The listing builds one solid part. Answer for the finished solid, in the listing's coordinates (mm). Face numbers are marked on the shaded views. A direction names the side the tool comes from. Round coordinates to 2 decimals unless told otherwise and drop trailing zeros. Order: outer loops, then holes, each group sorted by start corner. A loop starts at its lowest first (then second) coordinate and runs counter-clockwise, first axis right, second up. Notation, with made-up numbers: M 80.5,70.5 L 117.5,70.5 A27 cw 117.5,109.5 Z; hole C 12,44.25 d3. An arc over 180 degrees is marked long. Put each result on its own line as item: value. Start each with the question number.
1. The part is cut by section A-A (x = -8.5). Give the vertices of the cut face in (y, z).
2. The part is cut by section D-D (z = 2). Give the vertices of the cut face in (x, y), then the cut area to 3 significant figures.
3. Which of the six approach directions +Z, -Z, +X, -X, +Y, -Y give full straight-line access (tool end or side, diameter ignored) to the marked faces 1, 2, 3 and 4?
4. The part is cut by section C-C (x = -32). Give the vertices of the cut face in (y, z).
5. Each of these flat-tipped pins is pushed along its axis until it touches: pin 1 Ø6 at (x, y) = (-6.5, 62.5) entering from -Z; pin 2 Ø4.5 at (x, z) = (40, -12.5) entering from +Y; pin 3 Ø2 at (x, y) = (-1, -39) entering from -Z. Where does it stop, or does it pass through?
6. Consider line 1 (X direction, y = -82, z = 19); line 2 (Y direction, x = 36, z = 19.3); line 3 (Y direction, x = 15, z = 12.5). Determine where each line is inside the solid, lowest interval first.
7. The part is cut by section B-B (y = -38). Give the vertices of the cut face in (x, z), then the cut area to 3 significant figures.
8. The mould has two halves that part along Y. Classify the marked faces 5, 6 and 7: +Y half, -Y half, draft (parallel to the pull), parting line (faces both ways), or undercut.
from build123d import *

# Parameters (mm, degrees)
SKETCH1_W           = 75
SKETCH1_H           = 168
BOSS_EXTRUDE1_DEPTH = 20
BOSS_EXTRUDE2_DEPTH = 10
SKETCH3_W           = 6
SKETCH3_H           = 6
CUT_EXTRUDE2_DEPTH  = 39.37
SKETCH6_W           = 4
SKETCH6_H           = 5
CUT_EXTRUDE4_DEPTH  = 5
SKETCH7_W           = 69
SKETCH7_H           = 131
CUT_EXTRUDE5_DEPTH  = 16
SKETCH8_W           = 68.924591969
SKETCH8_H           = 27.4
CUT_EXTRUDE6_DEPTH  = 16
SKETCH9_W           = 16
SKETCH9_H           = 8
CUT_EXTRUDE7_DEPTH  = 16
SKETCH11_W          = 7.457157679
SKETCH11_H          = 6
CUT_EXTRUDE8_DEPTH  = 16
BOSS_EXTRUDE3_DEPTH = 10
FILLET4_START       = -3
FILLET4_DEPTH       = 6
FILLET4_START_2     = -50
FILLET4_2_DEPTH     = 131
FILLET5_R           = 2.2
SKETCH13_W          = 7
SKETCH13_H          = 18
BOSS_EXTRUDE4_DEPTH = 8
SKETCH14_W          = 2
SKETCH14_H          = 12.5
CUT_EXTRUDE9_DEPTH  = 99.169037889
SKETCH15_W          = 2
SKETCH15_H          = 12.5
CUT_EXTRUDE10_DEPTH = 99.169037889
SKETCH17_R          = 1
CUT_EXTRUDE11_DEPTH = 2


with BuildPart() as part:
    # Sketch1 → Boss-Extrude1 (new body)
    with BuildSketch(Plane.XY):
        Rectangle(SKETCH1_W, SKETCH1_H)
    extrude(amount=BOSS_EXTRUDE1_DEPTH)

    # Sketch7 → Cut-Extrude5 (cut)
    with BuildSketch(Plane.XY.offset(20)):
        with Locations((0, 15.5)):
            Rectangle(SKETCH7_W, SKETCH7_H)
    extrude(amount=-CUT_EXTRUDE5_DEPTH, mode=Mode.SUBTRACT)

    # Sketch8 → Cut-Extrude6 (cut)
    with BuildSketch(Plane.XY.offset(20)):
        with Locations((-0.037704015, -66.7)):
            Rectangle(SKETCH8_W, SKETCH8_H)
    extrude(amount=-CUT_EXTRUDE6_DEPTH, mode=Mode.SUBTRACT)

    # Sketch9 → Cut-Extrude7 (cut)
    with BuildSketch(Plane(origin=(0, -50, 0), x_dir=(1, 0, 0), z_dir=(0, 1, 0))):
        with Locations((-26.5, -12)):
            Rectangle(SKETCH9_W, SKETCH9_H)
        with Locations((26.5, -12)):
            Rectangle(SKETCH9_W, SKETCH9_H)
    extrude(amount=-CUT_EXTRUDE7_DEPTH, mode=Mode.SUBTRACT)


with BuildPart() as body_2:
    # Sketch2 → Boss-Extrude2 (new body)
    with BuildSketch(Plane(origin=(37.5, 0, 0), x_dir=(0, 0, -1), z_dir=(1, 0, 0))):
        Polygon((0, 5), (25.4, 5), (25.4, -5), (0, -5), (-20, -5), (-20, 5), align=None)
    extrude(amount=BOSS_EXTRUDE2_DEPTH)

    # Sketch3 → Cut-Extrude2 (cut)
    with BuildSketch(Plane.XY.offset(20)):
        with Locations((42.5, 0)):
            Rectangle(SKETCH3_W, SKETCH3_H)
    extrude(amount=-CUT_EXTRUDE2_DEPTH, mode=Mode.SUBTRACT)

    # Sketch6 → Cut-Extrude4 (cut)
    with BuildSketch(Plane(origin=(47.5, 0, 0), x_dir=(0, 0, -1), z_dir=(1, 0, 0))):
        with Locations((21.230369208, 0)):
            Rectangle(SKETCH6_W, SKETCH6_H)
    extrude(amount=-CUT_EXTRUDE4_DEPTH, mode=Mode.SUBTRACT)


with BuildPart() as cut_extrude8_tool:
    # Sketch11 → Cut-Extrude8 (new body)
    with BuildSketch(Plane.XY.offset(20)):
        with Locations((35.77142116, 0)):
            Rectangle(SKETCH11_W, SKETCH11_H)
    extrude(amount=-CUT_EXTRUDE8_DEPTH)


with BuildPart() as part_1:
    add(part.part)

    # Cut-Extrude8: cut by cut_extrude8_tool
    add(cut_extrude8_tool.part, mode=Mode.SUBTRACT)



with BuildPart() as body_2_1:
    add(body_2.part)

    # Cut-Extrude8: cut by cut_extrude8_tool
    add(cut_extrude8_tool.part, mode=Mode.SUBTRACT)


with BuildPart() as part_2:
    add(part_1.part)

    add(body_2_1.part)  # Boss-Extrude3 merges body 2
    # Sketch12 → Boss-Extrude3 (add)
    with BuildSketch(Plane.XZ.offset(5)):
        with BuildLine():
            Line((32.42, 0), (37.5, 0))
            Line((37.5, 0), (37.5, -5.08))
            ThreePointArc((37.5, -5.08), (36.012102448, -1.487897552), (32.42, 0))
        make_face()
    extrude(amount=-BOSS_EXTRUDE3_DEPTH)

    # Fillet4: read off the stored shape, not the designer's step
    # Fillet4 outline → Fillet4 (cut)
    with BuildSketch(Plane(origin=(0, 0, 0), x_dir=(1, 0, 0), z_dir=(0, 1, 0)).offset(FILLET4_START)):
        with BuildLine():
            Line((34.42, -4), (39.5, -4))
            Line((39.5, -4), (39.5, 1.08))
            ThreePointArc((39.5, 1.08), (38.012102448, -2.512102448), (34.42, -4))
        make_face()
    extrude(amount=FILLET4_DEPTH, mode=Mode.SUBTRACT)

    # Fillet4 2 outline → Fillet4 2 (cut)
    with BuildSketch(Plane(origin=(0, 0, 0), x_dir=(1, 0, 0), z_dir=(0, 1, 0)).offset(FILLET4_START_2)):
        with BuildLine():
            ThreePointArc((34.5, -3.99937004), (34.46000124, -3.999842507), (34.42, -4))
            Line((34.42, -4), (34.5, -4))
            Line((34.5, -4), (34.5, -3.99937004))
        make_face()
    extrude(amount=FILLET4_2_DEPTH, mode=Mode.SUBTRACT)

    # Fillet5
    fillet5_edges = [part_2.edges().sort_by_distance(p)[0] for p in [
        (42.5, 0, -19.37),
    ]]
    fillet(fillet5_edges, radius=FILLET5_R)

    # Sketch13 → Boss-Extrude4 (add)
    with BuildSketch(Plane(origin=(0, 0, 0), x_dir=(-1, 0, 0), z_dir=(0, 0, -1))):
        with Locations((0, 42)):
            Rectangle(SKETCH13_W, SKETCH13_H)
        with Locations((0, -42)):
            Rectangle(SKETCH13_W, SKETCH13_H)
    extrude(amount=BOSS_EXTRUDE4_DEPTH)

    # Sketch14 → Cut-Extrude9 (cut, through all)
    with BuildSketch(Plane(origin=(3.5, 0, 0), x_dir=(0, 0, -1), z_dir=(1, 0, 0))):
        with Locations((4, 42)):
            Rectangle(SKETCH14_W, SKETCH14_H)
    extrude(amount=-CUT_EXTRUDE9_DEPTH, mode=Mode.SUBTRACT)

    # Sketch15 → Cut-Extrude10 (cut, through all)
    with BuildSketch(Plane(origin=(3.5, 0, 0), x_dir=(0, 0, -1), z_dir=(1, 0, 0))):
        with Locations((4, -42)):
            Rectangle(SKETCH15_W, SKETCH15_H)
    extrude(amount=-CUT_EXTRUDE10_DEPTH, mode=Mode.SUBTRACT)

    # Sketch17 → Cut-Extrude11 (cut)
    with BuildSketch(Plane.XY.offset(20)):
        with Locations((-36.034629261, 82.534629261)):
            Circle(SKETCH17_R)
        with Locations((36, 82.5)):
            Circle(SKETCH17_R)
        with Locations((35.962295985, -82.2)):
            Circle(SKETCH17_R)
        with Locations((-36, -82.2)):
            Circle(SKETCH17_R)
    extrude(amount=-CUT_EXTRUDE11_DEPTH, mode=Mode.SUBTRACT)


solid = part_2.part
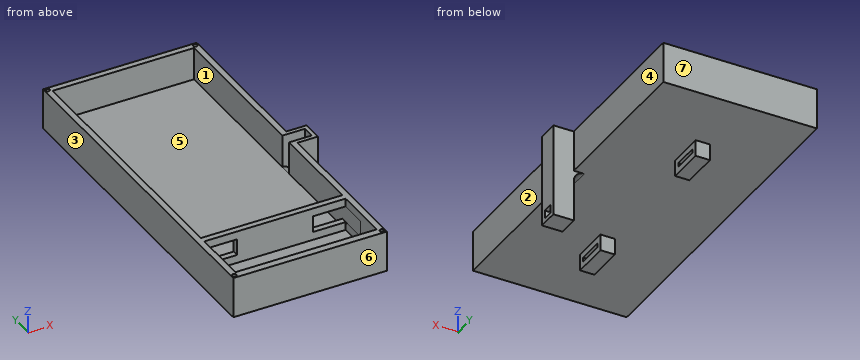
Resolved:
1. outline: M -84,0 L 84,0 L 84,20 L 81,20 L 81,4 L -50,4 L -50,20 L -53,20 L -53,4 L -80.4,4 L -80.4,20 L -84,20 Z
2. outline: M -37.5,-84 L 37.5,-84 L 37.5,-5 L 47.5,-5 L 47.5,5 L 37.5,5 L 37.5,84 L -37.5,84 Z; hole M 38.46,-3 L 45.5,-3 L 45.5,3 L 38.46,3 Z
2. area: 12,700 mm2
3. face 1: +Z
3. face 2: +Z, -Z, +X, -Y
3. face 3: +Z, -Z, -X, +Y, -Y
3. face 4: +Z, -Z, +X, +Y
4. outline: M -84,0 L 84,0 L 84,20 L 81,20 L 81,4 L -50,4 L -50,8 L -53,8 L -53,4 L -80.4,4 L -80.4,20 L -84,20 Z; M -53,16 L -50,16 L -50,20 L -53,20 Z
5. pin 1: z = 0
5. pin 2: y = 5
5. pin 3: z = -8
6. line 1: -37.5 to -36.98, -35.02 to 34.98, 36.94 to 37.5
6. line 2: -84 to -83.2, -81.2 to -3, 3 to 81.5, 83.5 to 84
6. line 3: -84 to -80.4, -53 to -50, 81 to 84
7. outline: M -37.5,0 L -3.5,0 L -3.5,-3 L 3.5,-3 L 3.5,0 L 37.5,0 L 37.5,20 L 34.5,20 L 34.5,4 A5.08 ccw 34.42,4 L -34.5,4 L -34.5,20 L -37.5,20 Z; M -3.5,-8 L 3.5,-8 L 3.5,-5 L -3.5,-5 Z
7. area: 438 mm2
8. face 5: undercut
8. face 6: -Y half
8. face 7: +Y half
